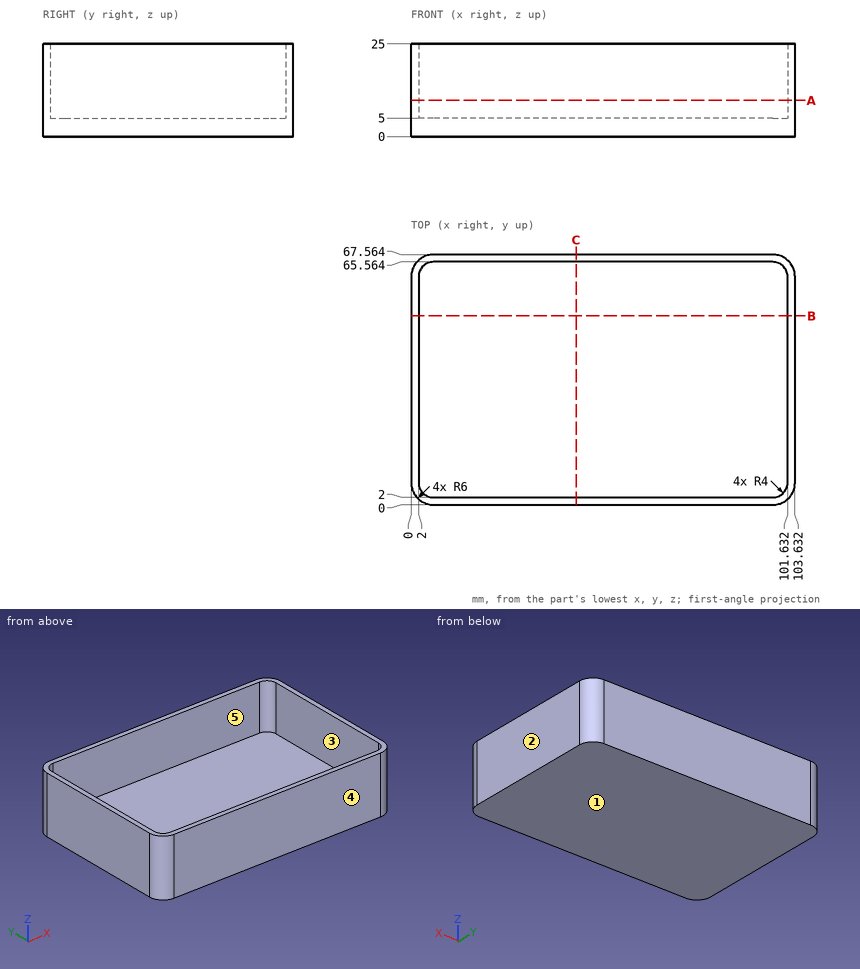
Source: three-view drawing plus pictorial views. Frame: mm from the lowest corner of the part. A direction names the side the tool comes from. Round coordinates to 2 decimals unless told otherwise and drop trailing zeros. Loops run counter-clockwise (first coordinate to the right, second up) from the corner with the lowest first, then second, coordinate; pieces in that order, holes last. Notation, with made-up numbers: (36.25, -4.5) - (44.25, -4.5) arc R14 ccw to (44.25, 16.5) - close; hole circle Ø9 at (26, 51). An arc over 180 degrees is marked (long way). Write each question's results on one line, items separated by ' | '. Start each with the question number.
1) Mould query, pull axis X, two halves, no side actions, for the marked faces 1, 2 and 3. Classes: released by +X, released by -X, zero draft, split by the parting line, or undercut.
2) Access query for the marked faces 4 and 5. Directions: +Z, -Z, +X, -X, +Y, -Y. A direction counts if a zero-diameter tool reaches every point of the face in a straight line with its end or side. Return the directions, or none.
3) Line query: probe 1 along Y at (x, z) = (82.5, 19.5); probe 2 along X at (y, z) = (37, 6.75); probe 3 along Z at (x, y) = (25, 58). Output: solid intervals per line, ascending. Write a range as [from, to].
4) Cut plane B-B on y = 51. Return loops of the section in (x, z).
5) Cut plane C-C on x = 44.5. Return loops of the section in (y, z), then the cut area to 3 significant figures.
6) Cut plane A-A on z = 9.75. Return loops of the section in (x, y), then the cut area to 3 significant figures.
Verdict:
1) face 1: zero draft | face 2: released by +X | face 3: undercut
2) face 4: +Z, -Z, +X, -X, -Y | face 5: +Z
3) probe 1: y = [0, 2], [65.56, 67.56] | probe 2: x = [0, 2], [101.63, 103.63] | probe 3: z = [0, 5]
4) outline: (0, 0) - (103.63, 0) - (103.63, 25) - (101.63, 25) - (101.63, 5) - (2, 5) - (2, 25) - (0, 25) - close
5) outline: (0, 0) - (67.56, 0) - (67.56, 25) - (65.56, 25) - (65.56, 5) - (2, 5) - (2, 25) - (0, 25) - close | area: 418 mm2
6) outline: (0, 6) arc R6 ccw to (6, 0) - (97.63, 0) arc R6 ccw to (103.63, 6) - (103.63, 61.56) arc R6 ccw to (97.63, 67.56) - (6, 67.56) arc R6 ccw to (0, 61.56) - close; hole (2, 6) arc R4 ccw to (6, 2) - (97.63, 2) arc R4 ccw to (101.63, 6) - (101.63, 61.56) arc R4 ccw to (97.63, 65.56) - (6, 65.56) arc R4 ccw to (2, 61.56) - close | area: 652 mm2
